from build123d import *

# Parameters (mm, degrees)
BOSS_EXTRUDE1_DEPTH            = 3
SKETCH2_W                      = 10
SKETCH2_H                      = 4.5
BOSS_EXTRUDE2_DEPTH            = 5
F_1_6_1_6_DIAMETER_HOLE1_D     = 1.6
F_1_6_1_6_DIAMETER_HOLE1_DEPTH = 4
F_1_6_1_6_DIAMETER_HOLE1_TIP   = 0.480688495
F_2_5_2_5_DIAMETER_HOLE1_D     = 2.5
F_2_5_2_5_DIAMETER_HOLE1_DEPTH = 4.5
M14_CLEARANCE_HOLE1_D          = 16.2
M14_CLEARANCE_HOLE1_DEPTH      = 3
FILLET1_R                      = 1.749999932


with BuildPart() as part:
    # Sketch1 → Boss-Extrude1 (new body)
    with BuildSketch(Plane.XZ):
        with BuildLine():
            Line((-5, 5.422252789), (-5, 0))
            Line((-5, 0), (5, 0))
            Line((5, 0), (5, 5.422252789))
            ThreePointArc((5, 5.422252789), (0, 23), (-5, 5.422252789))
        make_face()
    extrude(amount=-BOSS_EXTRUDE1_DEPTH)

    # Sketch2 → Boss-Extrude2 (add)
    with BuildSketch(Plane.XZ):
        with Locations((0, 2.25)):
            Rectangle(SKETCH2_W, SKETCH2_H)
    extrude(amount=BOSS_EXTRUDE2_DEPTH)

    # Ø1.6 (1.6) Diameter Hole1
    with Locations(Plane(origin=(0, 0, 0), x_dir=(-1, 0, 0), z_dir=(0, 0, -1))):
        with Locations((-3, 1)):
            Hole(F_1_6_1_6_DIAMETER_HOLE1_D / 2, depth=F_1_6_1_6_DIAMETER_HOLE1_DEPTH)
            with Locations((0, 0, -(F_1_6_1_6_DIAMETER_HOLE1_DEPTH + F_1_6_1_6_DIAMETER_HOLE1_TIP / 2))):  # 118° drill point
                Cone(0, F_1_6_1_6_DIAMETER_HOLE1_D / 2, F_1_6_1_6_DIAMETER_HOLE1_TIP, mode=Mode.SUBTRACT)

    # Ø2.5 (2.5) Diameter Hole1
    with Locations(Plane.XY.offset(4.5)):
        with Locations((-1.5, -2)):
            Hole(F_2_5_2_5_DIAMETER_HOLE1_D / 2, depth=F_2_5_2_5_DIAMETER_HOLE1_DEPTH)

    # M14 Clearance Hole1
    with Locations(Plane(origin=(0, 0, 0), x_dir=(-1, 0, 0), z_dir=(0, -1, 0))):
        with Locations((0, -13.5)):
            Hole(M14_CLEARANCE_HOLE1_D / 2, depth=M14_CLEARANCE_HOLE1_DEPTH)

    # Fillet1
    fillet1_edges = [part.edges().sort_by_distance(p)[0] for p in [
        (-5, 1.5, 5.422252789),
        (5, 1.5, 5.422252789),
    ]]
    fillet(fillet1_edges, radius=FILLET1_R)


solid = part.part
Input: part model. Units: mm. Frame: model coordinates. A direction names the side the tool comes from. Give positions to 0.01 mm unless a question says otherwise; leave off trailing zeros. Order: outer loops, then holes, each group sorted by start corner. A loop starts at its lowest first (then second) coordinate and runs counter-clockwise, first axis right, second up.
Q1. Draft query along Y for faces 1 (the cylindrical face through (3.763, 1.24, 2.028)), 2 (the flat face through (-8, 0, 16)), 3 (the flat face through (5, -1, 2)). Return one class per face: +Y half, -Y half, draft (parallel to the pull), parting line (faces both ways), or undercut.
Checked values:
face 1: undercut
face 2: -Y half
face 3: draft
Q2. Ray query, probe 1 along Y at (x, z) = (-1.5, 2.15); probe 2 along X at (y, z) = (1, 1.7); probe 3 along Y at (x, z) = (3, 2.25). Return the intervals inside material, ascending.
Checked values:
probe 1: y = -5 to -3.25, -0.75 to 3
probe 2: x = -5 to 2.2, 3.8 to 5
probe 3: y = -5 to 0.2, 1.8 to 3
Q3. Section B-B on x = 0. Output: boundary loops of the cut face in (y, z), and give its area (3 significant figures).
Checked values:
outline: (-5, 0) - (3, 0) - (3, 5.4) - (0, 5.4) - (0, 4.5) - (-5, 4.5) - close; (0, 21.6) - (3, 21.6) - (3, 23) - (0, 23) - close
area: 42.9 mm2
Q4. Contact query for flat-ended pins moving along their axis: pin 1 Ø3.5 at (y, z) = (-1.5, 1.5) entering from +X; pin 2 Ø1.4 at (y, z) = (-0.5, 1.5) entering from -X; pin 3 Ø3 at (x, y) = (7.5, 0.5) entering from +Z; pin 4 Ø5.5 at (x, z) = (-1.5, 17) entering from -Y. Output: stop coordinate, or through.
Checked values:
pin 1: stops at x = 5
pin 2: stops at x = -5
pin 3: stops at z = 20.87
pin 4: passes through
Q5. Section C-C on z = 13.5. Output: boundary loops of the cut face in (x, y).
Checked values:
outline: (-9.5, 0) - (-8.1, 0) - (-8.1, 3) - (-9.5, 3) - close; (8.1, 0) - (9.5, 0) - (9.5, 3) - (8.1, 3) - close
Q6. Section D-D on z = 2. Output: boundary loops of the cut face in (x, y), and give its area (3 significant figures).
Checked values:
outline: (-5, -5) - (5, -5) - (5, 3) - (-5, 3) - close; hole circle Ø2.5 at (-1.5, -2); hole circle Ø1.6 at (3, 1)
area: 73.1 mm2
Q7. Section A-A on y = -2.75. Output: boundary loops of the cut face in (x, z).
Checked values:
outline: (-5, 0) - (-2.5, 0) - (-2.5, 4.5) - (-5, 4.5) - close; (-0.5, 0) - (5, 0) - (5, 4.5) - (-0.5, 4.5) - close
Q8. Set-up query: faces 4 (the flat face through (0, -2, 4.5)), 5 (the flat face through (-5, -1, 2)), 6 (the flat face through (-1, 3, 5)). Return all of +Z, -Z, +X, -X, +Y, -Y with unobstructed straight access to the full face (end or side cutting, diameter ignored); none if empty.
Checked values:
face 4: +Z, +X, -X, -Y
face 5: -Z, -X, +Y, -Y
face 6: +Z, -Z, +X, -X, +Y
